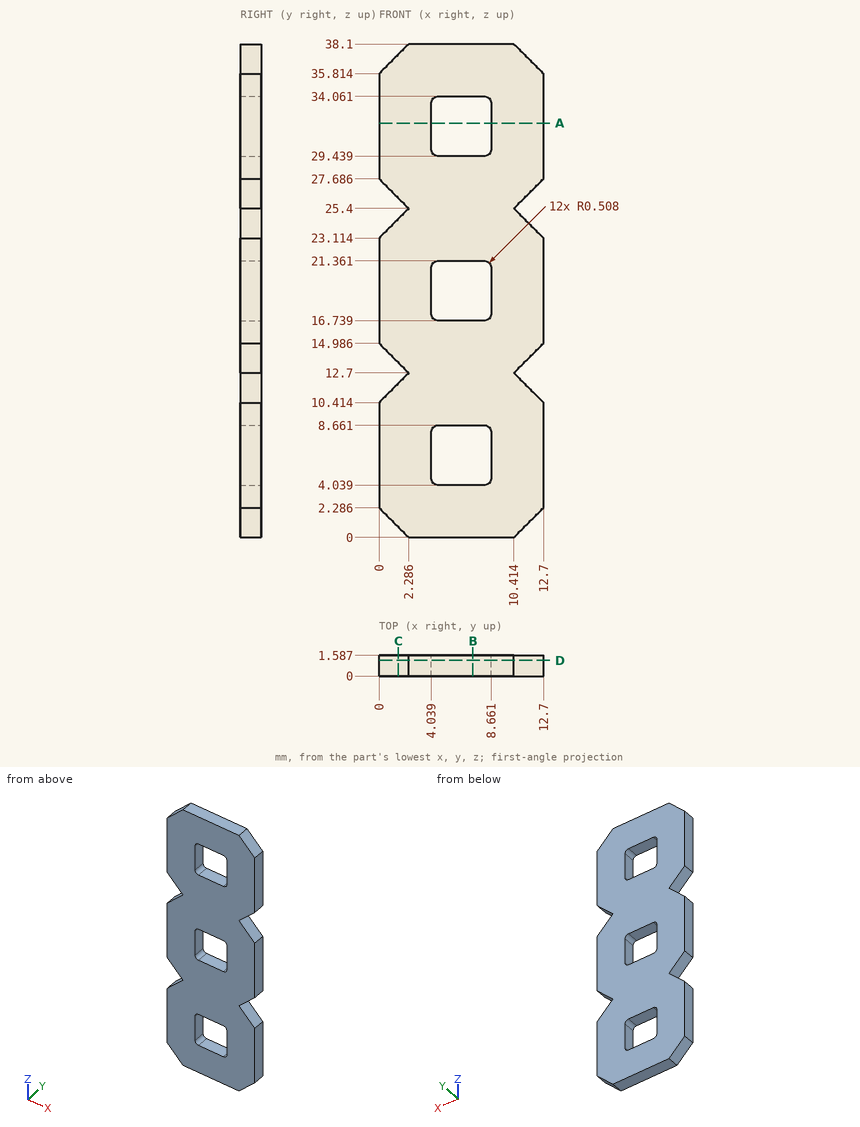
Can you work these out from the drawing? Everything is in mm from the part's minimum corner. Round coordinates to 2 decimals unless told otherwise and drop trailing zeros. Loops run counter-clockwise (first coordinate to the right, second up) from the corner with the lowest first, then second, coordinate; pieces in that order, holes last. Notation, with made-up numbers: M 87.25,73.5 L 119.25,73.5 A3 ccw 119.25,78.5 Z; hole C 87,-38 d9. An arc over 180 degrees is marked long. Answer in a Markdown table with one row per item.
1. Please list where these lines run through material, in increasing order: line 1 (Z direction, x = 4.5, y = 1.25); line 2 (X direction, y = 1, z = 30.5); line 3 (Z direction, x = 4.25, y = 1.25) (1 decimal). Write a range as from..to.
Established:
| item | result |
|---|---|
| line 1 | 0..4.04, 8.66..16.74, 21.36..29.44, 34.06..38.1 |
| line 2 | 0..4.04, 8.66..12.7 |
| line 3 | 0..4.1, 8.6..16.8, 21.3..29.5, 34..38.1 |
2. If we section it at C-C, the plane x = 1.5: Please give me the cut outline in (y, z) (1 decimal).
Established:
| item | result |
|---|---|
| outline | M 0,0.8 L 1.6,0.8 L 1.6,11.9 L 0,11.9 Z; M 0,13.5 L 1.6,13.5 L 1.6,24.6 L 0,24.6 Z; M 0,26.2 L 1.6,26.2 L 1.6,37.3 L 0,37.3 Z |
3. I'm going to push a flat-ended pin straight in: pin 1 Ø0.8 at (x, y) = (6, 0.5) entering from -Z. Where does the tip first touch, or does it pass through?
Established:
| item | result |
|---|---|
| pin 1 | z = 0 |
4. If we section it at D-D, the plane y = 1.2: Give the number of separate pieces and of enclosed holes in the cut face, plus the area to 3 significant figures.
Established:
| item | result |
|---|---|
| separate pieces | 1 |
| enclosed holes | 3 |
| area | 389 mm² |
5. If we section it at B-B, the plane x = 7.25: Please give me the cut outline in (y, z).
Established:
| item | result |
|---|---|
| outline | M 0,0 L 1.59,0 L 1.59,4.04 L 0,4.04 Z; M 0,8.66 L 1.59,8.66 L 1.59,16.74 L 0,16.74 Z; M 0,21.36 L 1.59,21.36 L 1.59,29.44 L 0,29.44 Z; M 0,34.06 L 1.59,34.06 L 1.59,38.1 L 0,38.1 Z |
6. If we section it at A-A, the plane z = 32: Please give me the cut outline in (x, y).
Established:
| item | result |
|---|---|
| outline | M 0,0 L 4.04,0 L 4.04,1.59 L 0,1.59 Z; M 8.66,0 L 12.7,0 L 12.7,1.59 L 8.66,1.59 Z |
